from build123d import *

# Parameters (mm, degrees)
SKETCH1_W           = 50
SKETCH1_H           = 25
BOSS_EXTRUDE2_DEPTH = 100
SKETCH1_4_W         = 10
SKETCH1_4_H         = 25
BOSS_EXTRUDE3_DEPTH = 65
BOSS_EXTRUDE4_DEPTH = 25
BOSS_EXTRUDE5_DEPTH = 50
SKETCH4_R           = 12.5
CUT_EXTRUDE1_DEPTH  = 56
CUT_EXTRUDE2_DEPTH  = 56


with BuildPart() as part:
    # Sketch1 → Boss-Extrude2 (new body)
    with BuildSketch(Plane.XY):
        with Locations((-60.137096774, -53.32358871)):
            Rectangle(SKETCH1_W, SKETCH1_H)
    extrude(amount=BOSS_EXTRUDE2_DEPTH)

    # Sketch1_4 → Boss-Extrude3 (add)
    with BuildSketch(Plane.XY):
        with Locations((-80.137096774, -28.32358871)):
            Rectangle(SKETCH1_4_W, SKETCH1_4_H)
        with Locations((-40.137096774, -28.32358871)):
            Rectangle(SKETCH1_4_W, SKETCH1_4_H)
    extrude(amount=BOSS_EXTRUDE3_DEPTH)

    # Sketch1_5 → Boss-Extrude4 (add)
    with BuildSketch(Plane.XY):
        with BuildLine():
            Line((-75.137096774, -15.82358871), (-75.137096774, -40.82358871))
            Line((-75.137096774, -40.82358871), (-45.137096774, -40.82358871))
            Line((-45.137096774, -40.82358871), (-45.137096774, -15.82358871))
            Line((-45.137096774, -15.82358871), (-35.137096774, -15.82358871))
            Line((-35.137096774, -15.82358871), (-35.137096774, 34.17641129))
            ThreePointArc((-35.137096774, 34.17641129), (-60.137096774, 9.17641129), (-85.137096774, 34.17641129))
            Line((-85.137096774, 34.17641129), (-85.137096774, -15.82358871))
            Line((-85.137096774, -15.82358871), (-75.137096774, -15.82358871))
        make_face()
    extrude(amount=BOSS_EXTRUDE4_DEPTH)

    # Sketch1_6 → Boss-Extrude5 (add)
    with BuildSketch(Plane.XY):
        with BuildLine():
            ThreePointArc((-75.137096774, 34.17641129), (-60.137096774, 19.17641129), (-45.137096774, 34.17641129))
            Line((-45.137096774, 34.17641129), (-35.137096774, 34.17641129))
            ThreePointArc((-35.137096774, 34.17641129), (-60.137096774, 9.17641129), (-85.137096774, 34.17641129))
            Line((-85.137096774, 34.17641129), (-75.137096774, 34.17641129))
        make_face()
    extrude(amount=BOSS_EXTRUDE5_DEPTH)

    # Sketch4 → Cut-Extrude1 (cut)
    with BuildSketch(Plane(origin=(0, -40.82358871, 0), x_dir=(1, 0, 0), z_dir=(0, 1, 0))):
        with Locations((-60.137096774, -80)):
            Circle(SKETCH4_R)
        with BuildLine():
            Line((-35.137096774, -100), (-35.137096774, -82.5))
            Line((-35.137096774, -82.5), (-40.293961941, -82.5))
            ThreePointArc((-40.293961941, -82.5), (-46.908340219, -95), (-60.137096774, -100))
            Line((-60.137096774, -100), (-35.137096774, -100))
        make_face()
        with BuildLine():
            Line((-85.137096774, -100), (-60.137096774, -100))
            ThreePointArc((-60.137096774, -100), (-73.36585333, -95), (-79.980231607, -82.5))
            Line((-79.980231607, -82.5), (-85.137096774, -82.5))
            Line((-85.137096774, -82.5), (-85.137096774, -100))
        make_face()
    extrude(amount=-CUT_EXTRUDE1_DEPTH, mode=Mode.SUBTRACT)

    # Sketch7 → Cut-Extrude2 (cut)
    with BuildSketch(Plane(origin=(-35.137096774, 0, 0), x_dir=(0, 0, -1), z_dir=(1, 0, 0))):
        Polygon((-65, -15.82358871), (-65, -40.82358871), (-43.333333333, -15.82358871), align=None)
    extrude(amount=-CUT_EXTRUDE2_DEPTH, mode=Mode.SUBTRACT)


solid = part.part
Work out the finished part from the listing and answer in its coordinate system (mm). A direction names the side the tool comes from. Coordinates: 2 decimals unless noted, no trailing zeros. Loops run counter-clockwise (first coordinate to the right, second up) from the corner with the lowest first, then second, coordinate; pieces in that order, holes last. Notation, with made-up numbers: M -33,41 L 15,41 A19 cw 15,52 Z; hole C -4.75,55 d5. An arc over 180 degrees is marked long. Answer in a Markdown table with one row per item. Add a question column.
1. A tool of negligible diameter and unlimited length cuts with its end or side. For faces 5 (the flat face through (-38, -53, 82.5)), 6 (the flat face through (-40, -15.824, 34)), 7 (the flat face through (-60, 19, 50)), 8 (the flat face through (-45.137, -31, 40)), 9 (the flat face through (-83, -53, 82.5)), from which of +Z, -Z, +X, -X, +Y, -Y can it reach the whole face along a straight path? Write none if from no direction.
2. Consider L1, parallel to X at y = -58, z = 80; L2, parallel to X at y = -24, z = 49.5; L3, parallel to Z at x = -60.5, y = 5. Determine where each line is inside the solid, lowest interval first.
3. Find section D-D, the plane y = 27. Write down the section's boundary in (x, z), then the cut area to 3 significant figures.
4. The mould has two halves that part along Y. Classify faces 1 (the flat face through (-60, -65.824, 38)), 2 (the flat face through (-85.137, -26, 32)), 3 (the flat face through (-80.07, -28.5, 54.32)), 4 (the flat face through (-40.07, -28.5, 54.32)): pulls with the +Y half, pulls with the -Y half, needs draft (parallel to the pull), parting line crosses it, or undercut.
5. Find section A-A, the plane z = 80. Write down the section's boundary in (x, y), then the cut area to 3 significant figures.
6. Find section B-B, the plane y = -55.5. Write down the section's boundary in (x, z).
7. Find section C-C, the plane x = -62. Write down the section's boundary in (y, z).
8. Flat-ended cylindrical pins translate along their axes: P1, Ø8, axis at x = -58, z = 65, coming from the +Y side; P2, Ø25, axis at x = -59.5, y = -3.5, coming from the +Z side; P3, Ø4, axis at x = -36.5, y = -58.5, coming from the +Z side. Find the tip coordinate at first contact, or state that the pin passes through.
Reported:
| question | item | result |
|---|---|---|
| 1 | face 5 | +Z, +X, +Y, -Y |
| 1 | face 6 | +Z, +X, -X |
| 1 | face 7 | +Z, +X, -X, +Y |
| 1 | face 8 | +Z |
| 1 | face 9 | +Z, -X, +Y, -Y |
| 2 | L1 | x = -85.14 to -72.64, -47.64 to -35.14 |
| 2 | L2 | x = -85.14 to -75.14, -45.14 to -35.14 |
| 2 | L3 | z = 0 to 25 |
| 3 | outline | M -85.14,0 L -73.31,0 L -73.31,50 L -84.08,50 L -84.08,25 L -85.14,25 Z; M -46.97,0 L -35.14,0 L -35.14,25 L -36.19,25 L -36.19,50 L -46.97,50 Z |
| 3 | area | 1,130 mm^2 |
| 4 | face 1 | pulls with the -Y half |
| 4 | face 2 | needs draft |
| 4 | face 3 | undercut |
| 4 | face 4 | undercut |
| 5 | outline | M -85.14,-65.82 L -72.64,-65.82 L -72.64,-40.82 L -85.14,-40.82 Z; M -47.64,-65.82 L -35.14,-65.82 L -35.14,-40.82 L -47.64,-40.82 Z |
| 5 | area | 625 mm^2 |
| 6 | outline | M -85.14,0 L -35.14,0 L -35.14,82.5 L -40.29,82.5 A20 ccw -79.98,82.5 L -85.14,82.5 Z; hole C -60.14,80 d25 |
| 7 | outline | M -65.82,0 L 19.29,0 L 19.29,50 L 9.25,50 L 9.25,25 L -40.82,25 L -40.82,67.64 L -65.82,67.64 Z; M -65.82,92.36 L -40.82,92.36 L -40.82,99.91 L -65.82,99.91 Z |
| 8 | P1 | stops at y = -40.82 |
| 8 | P2 | stops at z = 25 |
| 8 | P3 | stops at z = 82.5 |
